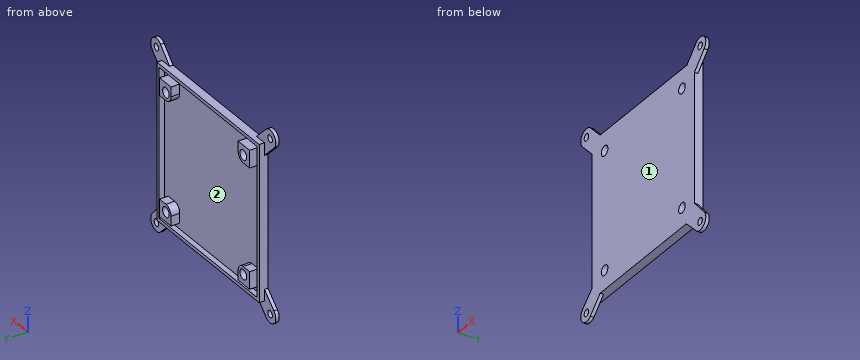
```python
from build123d import *

# Parameters (mm, degrees)
SKETCH1_W            = 90
SKETCH1_H            = 90
SKETCH1_W_2          = 86
SKETCH1_H_2          = 86
BOSS_EXTRUDE1_DEPTH  = 5
BOSS_EXTRUDE2_DEPTH  = 2
SKETCH1_9_R          = 2.9
BOSS_EXTRUDE11_DEPTH = 7
SKETCH1_10_W         = 59
SKETCH1_10_H         = 2.08
SKETCH1_10_W_2       = 2.08
SKETCH1_10_H_2       = 59
BOSS_EXTRUDE12_DEPTH = 2
SKETCH2_R            = 2
BOSS_EXTRUDE13_DEPTH = 2


with BuildPart() as part:
    # Sketch1 → Boss-Extrude1 (new body)
    with BuildSketch(Plane(origin=(0, 0, 0), x_dir=(1, 0, 0), z_dir=(0, 1, 0))):
        with Locations((-213.560874466, -146.147776914)):
            Rectangle(SKETCH1_W, SKETCH1_H)
        with Locations((-213.560874466, -146.147776914)):
            Rectangle(SKETCH1_W_2, SKETCH1_H_2, mode=Mode.SUBTRACT)
    extrude(amount=BOSS_EXTRUDE1_DEPTH)

    # Sketch1_3 → Boss-Extrude2 (add)
    with BuildSketch(Plane(origin=(0, 0, 0), x_dir=(1, 0, 0), z_dir=(0, 1, 0))):
        Polygon((-173.980874466, -189.147776914), (-170.560874466, -189.147776914), (-170.560874466, -103.147776914), (-256.560874466, -103.147776914), (-256.560874466, -189.147776914), align=None)
        Polygon((-173.980874466, -175.647776914), (-173.980874466, -185.727776914), (-176.060874466, -185.727776914), (-184.060874466, -185.727776914), (-243.060874466, -185.727776914), (-253.140874466, -185.727776914), (-253.140874466, -175.647776914), (-253.140874466, -116.647776914), (-253.140874466, -106.567776914), (-243.060874466, -106.567776914), (-184.060874466, -106.567776914), (-173.980874466, -106.567776914), (-173.980874466, -116.647776914), align=None, mode=Mode.SUBTRACT)
    extrude(amount=BOSS_EXTRUDE2_DEPTH)

    # Sketch1_9 → Boss-Extrude11 (add)
    # profile 1 of 4: a face of its own
    with BuildSketch(Plane(origin=(0, 0, 0), x_dir=(1, 0, 0), z_dir=(0, 1, 0))):
        with BuildLine():
            Line((-173.980874466, -185.727776914), (-173.980874466, -175.647776914))
            Line((-173.980874466, -175.647776914), (-179.560874466, -175.647776914))
            ThreePointArc((-179.560874466, -175.647776914), (-182.742854981, -176.965796398), (-184.060874466, -180.147776914))
            Line((-184.060874466, -180.147776914), (-184.060874466, -185.727776914))
            Line((-184.060874466, -185.727776914), (-173.980874466, -185.727776914))
        make_face()
        with Locations(Location((-179.560874466, -180.147776914, 0), (0, 0, 270))):
            Circle(SKETCH1_9_R, mode=Mode.SUBTRACT)
    # profile 2 of 4: a face of its own
    with BuildSketch(Plane(origin=(0, 0, 0), x_dir=(1, 0, 0), z_dir=(0, 1, 0))):
        with BuildLine():
            Line((-173.980874466, -116.647776914), (-173.980874466, -106.567776914))
            Line((-173.980874466, -106.567776914), (-184.060874466, -106.567776914))
            Line((-184.060874466, -106.567776914), (-184.060874466, -112.147776914))
            ThreePointArc((-184.060874466, -112.147776914), (-182.742854981, -115.329757429), (-179.560874466, -116.647776914))
            Line((-179.560874466, -116.647776914), (-173.980874466, -116.647776914))
        make_face()
        with Locations(Location((-179.560874466, -112.147776914, 0), (0, 0, 270))):
            Circle(SKETCH1_9_R, mode=Mode.SUBTRACT)
    # profile 3 of 4: a face of its own
    with BuildSketch(Plane(origin=(0, 0, 0), x_dir=(1, 0, 0), z_dir=(0, 1, 0))):
        with BuildLine():
            Line((-253.140874466, -185.727776914), (-243.060874466, -185.727776914))
            Line((-243.060874466, -185.727776914), (-243.060874466, -180.147776914))
            ThreePointArc((-243.060874466, -180.147776914), (-244.378893951, -176.965796398), (-247.560874466, -175.647776914))
            Line((-247.560874466, -175.647776914), (-253.140874466, -175.647776914))
            Line((-253.140874466, -175.647776914), (-253.140874466, -185.727776914))
        make_face()
        with Locations(Location((-247.560874466, -180.147776914, 0), (0, 0, 270))):
            Circle(SKETCH1_9_R, mode=Mode.SUBTRACT)
    # profile 4 of 4: a face of its own
    with BuildSketch(Plane(origin=(0, 0, 0), x_dir=(1, 0, 0), z_dir=(0, 1, 0))):
        with BuildLine():
            Line((-243.060874466, -106.567776914), (-253.140874466, -106.567776914))
            Line((-253.140874466, -106.567776914), (-253.140874466, -116.647776914))
            Line((-253.140874466, -116.647776914), (-247.560874466, -116.647776914))
            ThreePointArc((-247.560874466, -116.647776914), (-244.378893951, -115.329757429), (-243.060874466, -112.147776914))
            Line((-243.060874466, -112.147776914), (-243.060874466, -106.567776914))
        make_face()
        with Locations(Location((-247.560874466, -112.147776914, 0), (0, 0, 270))):
            Circle(SKETCH1_9_R, mode=Mode.SUBTRACT)
    extrude(amount=BOSS_EXTRUDE11_DEPTH)

    # Sketch1_10 → Boss-Extrude12 (add)
    with BuildSketch(Plane(origin=(0, 0, 0), x_dir=(1, 0, 0), z_dir=(0, 1, 0))):
        with Locations((-213.560874466, -107.607776914)):
            Rectangle(SKETCH1_10_W, SKETCH1_10_H)
        with Locations((-175.020874466, -146.147776914)):
            Rectangle(SKETCH1_10_W_2, SKETCH1_10_H_2)
        with Locations((-213.560874466, -184.687776914)):
            Rectangle(SKETCH1_10_W, SKETCH1_10_H)
        with Locations((-252.100874466, -146.147776914)):
            Rectangle(SKETCH1_10_W_2, SKETCH1_10_H_2)
        with BuildLine():
            Line((-179.560874466, -175.647776914), (-176.060874466, -175.647776914))
            Line((-176.060874466, -175.647776914), (-176.060874466, -116.647776914))
            Line((-176.060874466, -116.647776914), (-179.560874466, -116.647776914))
            ThreePointArc((-179.560874466, -116.647776914), (-182.742854981, -115.329757429), (-184.060874466, -112.147776914))
            Line((-184.060874466, -112.147776914), (-184.060874466, -108.647776914))
            Line((-184.060874466, -108.647776914), (-243.060874466, -108.647776914))
            Line((-243.060874466, -108.647776914), (-243.060874466, -112.147776914))
            ThreePointArc((-243.060874466, -112.147776914), (-244.378893951, -115.329757429), (-247.560874466, -116.647776914))
            Line((-247.560874466, -116.647776914), (-251.060874466, -116.647776914))
            Line((-251.060874466, -116.647776914), (-251.060874466, -175.647776914))
            Line((-251.060874466, -175.647776914), (-247.560874466, -175.647776914))
            ThreePointArc((-247.560874466, -175.647776914), (-244.378893951, -176.965796398), (-243.060874466, -180.147776914))
            Line((-243.060874466, -180.147776914), (-243.060874466, -183.647776914))
            Line((-243.060874466, -183.647776914), (-184.060874466, -183.647776914))
            Line((-184.060874466, -183.647776914), (-184.060874466, -180.147776914))
            ThreePointArc((-184.060874466, -180.147776914), (-182.742854981, -176.965796398), (-179.560874466, -175.647776914))
        make_face()
    extrude(amount=BOSS_EXTRUDE12_DEPTH)

    # Sketch2 → Boss-Extrude13 (add)
    # profile 1 of 4: a face of its own
    with BuildSketch(Plane.XZ):
        with BuildLine():
            Line((-159.906154646, 99.555585085), (-168.560874466, 109.105835649))
            Line((-168.560874466, 109.105835649), (-168.560874466, 101.147776914))
            Line((-168.560874466, 101.147776914), (-175.623402457, 101.147776914))
            Line((-175.623402457, 101.147776914), (-167.316099349, 92.840473806))
            ThreePointArc((-167.316099349, 92.840473806), (-160.253571358, 92.493057094), (-159.906154646, 99.555585085))
        make_face()
        with Locations(Location((-163.611126998, 96.198029445, 0), (0, 0, 270))):
            Circle(SKETCH2_R, mode=Mode.SUBTRACT)
    # profile 2 of 4: a face of its own
    with BuildSketch(Plane.XZ):
        with BuildLine():
            Line((-266.92065329, 99.854761067), (-258.560874466, 107.650550002))
            Line((-258.560874466, 107.650550002), (-258.560874466, 101.147776914))
            Line((-258.560874466, 101.147776914), (-251.494111489, 101.147776914))
            Line((-251.494111489, 101.147776914), (-260.100590579, 92.541297823))
            ThreePointArc((-260.100590579, 92.541297823), (-267.167353556, 92.78799809), (-266.92065329, 99.854761067))
        make_face()
        with Locations(Location((-263.510621934, 96.198029445, 0), (0, 0, 270))):
            Circle(SKETCH2_R, mode=Mode.SUBTRACT)
    # profile 3 of 4: a face of its own
    with BuildSketch(Plane.XZ):
        with BuildLine():
            Line((-259.953166758, 199.611000249), (-251.594570664, 191.147776914))
            Line((-251.594570664, 191.147776914), (-258.560874466, 191.147776914))
            Line((-258.560874466, 191.147776914), (-258.560874466, 183.970358473))
            Line((-258.560874466, 183.970358473), (-267.068077111, 192.584048515))
            ThreePointArc((-267.068077111, 192.584048515), (-267.024097801, 199.654979559), (-259.953166758, 199.611000249))
        make_face()
        with Locations(Location((-263.510621934, 196.097524382, 0), (0, 0, 270))):
            Circle(SKETCH2_R, mode=Mode.SUBTRACT)
    # profile 4 of 4: a face of its own
    with BuildSketch(Plane.XZ):
        with BuildLine():
            Line((-167.239177795, 199.538054488), (-175.195792575, 191.147776914))
            Line((-175.195792575, 191.147776914), (-168.560874466, 191.147776914))
            Line((-168.560874466, 191.147776914), (-168.560874466, 183.611676585))
            Line((-168.560874466, 183.611676585), (-159.983076201, 192.656994276))
            ThreePointArc((-159.983076201, 192.656994276), (-160.170596891, 199.725575179), (-167.239177795, 199.538054488))
        make_face()
        with Locations(Location((-163.611126998, 196.097524382, 0), (0, 0, 270))):
            Circle(SKETCH2_R, mode=Mode.SUBTRACT)
    extrude(amount=-BOSS_EXTRUDE13_DEPTH)


solid = part.part
```
The model under review builds one solid part; all positions refer to its coordinate system, in mm. Face numbers are marked on the shaded views. Round coordinates to 2 decimals unless told otherwise and drop trailing zeros. Loops run counter-clockwise (first coordinate to the right, second up) from the corner with the lowest first, then second, coordinate; pieces in that order, holes last. Notation, with made-up numbers: (77, 31) -> (108, 31) arc R34 ccw to (108, 64) -> close; hole circle Ø4 at (43, -16). An arc over 180 degrees is marked (long way). Answer as a JSON object with one key per item and string values. Group by question number.
1) For pin 1 Ø1 at (y, z) = (1, 131) entering from -X; pin 2 Ø4.5 at (x, z) = (-179.56, 112.15) entering from -Y; pin 3 Ø3.5 at (x, y) = (-227.5, 3.5) entering from +Z; pin 4 Ø10 at (x, z) = (-235.5, 151) entering from +Y, all flat-tipped, find the tip position at first contact; note any pin that passes through.
2) We need section B-B on z = 148. Write out the cut boundary in (x, y).
3) For line 1 (Z direction, x = -213, y = 3.75); line 2 (X direction, y = 3.25, z = 147.5); line 3 (X direction, y = 6.5, z = 184), list the stretches that pass through material, from the lowest coordinate up. Write a range as [from, to].
4) We need section A-A on x = -211.5. Write out the cut boundary in (y, z).
5) Mouldability with a two-part tool opening along Z and no side actions: class the marked faces 1 and 2 as released by +Z, released by -Z, zero draft, split by the parting line, or undercut.
Result set:
{
 "1": {"pin 1": "x = -258.56", "pin 2": "through", "pin 3": "z = 191.15", "pin 4": "y = 2"},
 "2": {"outline": "(-258.56, 0) -> (-168.56, 0) -> (-168.56, 5) -> (-170.56, 5) -> (-170.56, 2) -> (-256.56, 2) -> (-256.56, 5) -> (-258.56, 5) -> close"},
 "3": {"line 1": "[101.15, 103.15], [189.15, 191.15]", "line 2": "[-258.56, -256.56], [-170.56, -168.56]", "line 3": "[-253.14, -243.06], [-184.06, -173.98]"},
 "4": {"outline": "(0, 101.15) -> (5, 101.15) -> (5, 103.15) -> (2, 103.15) -> (2, 189.15) -> (5, 189.15) -> (5, 191.15) -> (0, 191.15) -> close"},
 "5": {"face 1": "zero draft", "face 2": "undercut"}
}
